The drawing under review shows one solid part. Ordinate dimensions are in mm from its lowest x, y, z. A direction names the side the tool comes from. Coordinates: 2 decimals unless noted, no trailing zeros. Write each loop counter-clockwise with the first axis right and the second up, starting at its lowest first coordinate (ties: lowest second). Pieces come first, ordered by that corner, then holes.
1) Add section C-C, the plane x = 77. State the section outline as (y, z) points.
2) For P1, Ø25, axis at x = 78, y = 67.5, coming from the +Z side; P2, Ø6, axis at y = 22.5, z = 57.5, coming from the +X side, all flat-tipped, find the tip position at first contact; note any pin that passes through.
3) Machinability: for the marked faces 1 and 2, which of the approach directions +Z, -Z, +X, -X, +Y, -Y give a long, thin tool a straight path to every point of the face, cutting with its end or side? Answer none if there is none.
4) For line 1 (Z direction, x = 70, y = 19.5); line 2 (X direction, y = 78, z = 66), list the stretches that pass through material, from the lowest coordinate up.
5) Add section B-B, the plane z = 90.5. State the section outline as (x, y) points, then the cut area to 3 significant figures.
6) Add section A-A, the plane y = 31. State the section outline as (x, z) points.
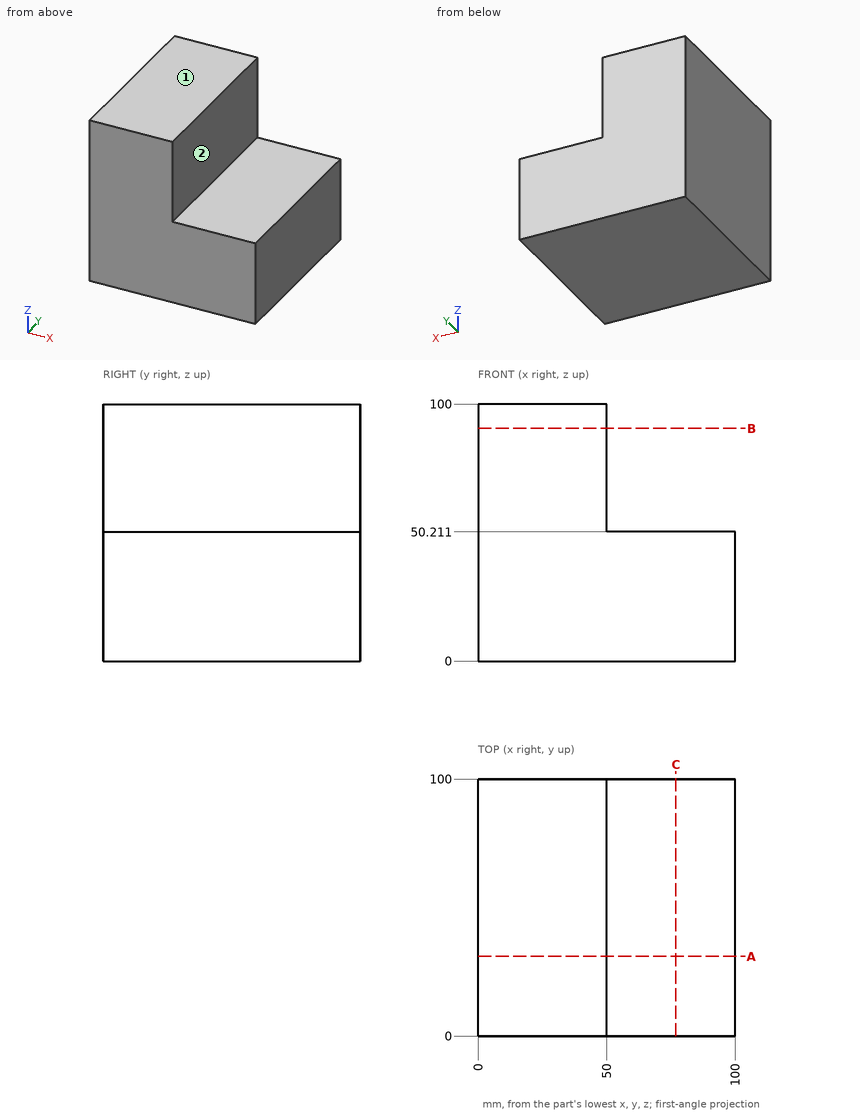
Geometry results:
1. outline: (0, 0) - (100, 0) - (100, 50.21) - (0, 50.21) - close
2. P1: stops at z = 50.21
2. P2: stops at x = 50
3. face 1: +Z, +X, -X, +Y, -Y
3. face 2: +Z, +X, +Y, -Y
4. line 1: z = 0 to 50.21
4. line 2: x = 0 to 50
5. outline: (0, 0) - (50, 0) - (50, 100) - (0, 100) - close
5. area: 5,000 mm2
6. outline: (0, 0) - (100, 0) - (100, 50.21) - (50, 50.21) - (50, 100) - (0, 100) - close
